```python
from build123d import *

# Parameters (mm, degrees)
SKETCH_1_R          = 1.6
EXTRUDE_1_DEPTH     = 3
CUT_EXTRUDE_1_DEPTH = 4
SKETCH_4_R          = 43
CUT_EXTRUDE_2_DEPTH = 10
FILLET_1_R          = 2


with BuildPart() as part:
    # 草图1 → 凸台-拉伸1 (new body)
    with BuildSketch(Plane.XY):
        with BuildLine():
            Line((45.024979201, 5), (65, 5))
            Line((65, 5), (65, -5))
            Line((65, -5), (50, -20))
            Line((50, -20), (10, -20))
            Line((10, -20), (-5, -5))
            Line((-5, -5), (-5, 5))
            Line((-5, 5), (14.975020799, 5))
            ThreePointArc((14.975020799, 5), (30, 1.5), (45.024979201, 5))
        make_face()
        with Locations((60, 0)):
            Circle(SKETCH_1_R, mode=Mode.SUBTRACT)
        Circle(SKETCH_1_R, mode=Mode.SUBTRACT)
    extrude(amount=EXTRUDE_1_DEPTH)

    # 草图3 → 切除-拉伸1 (cut, through all)
    with BuildSketch(Plane(origin=(0, 0, 0), x_dir=(-1, 0, 0), z_dir=(0, 0, -1))):
        Polygon((-25, -15.464816242), (-15, -15.464816242), (-6.245134561, -2.961572616), align=None)
        Polygon((-53.754865439, -2.961572616), (-35, -15.464816242), (-45, -15.464816242), align=None)
    extrude(amount=-CUT_EXTRUDE_1_DEPTH, mode=Mode.SUBTRACT)

    # 草图4 → 切除-拉伸2 (cut)
    with BuildSketch(Plane.XY.offset(3)):
        with Locations((30, 35.5)):
            Circle(SKETCH_4_R)
    extrude(amount=-CUT_EXTRUDE_2_DEPTH, mode=Mode.SUBTRACT)

    # 圆角1
    fillet_1_edges = [part.edges().sort_by_distance(p)[0] for p in [
        (50, -20, 1.5),
        (10, -20, 1.5),
        (-5, -5, 1.5),
        (-5, 5, 1.5),
        (65, 5, 1.5),
        (65, -5, 1.5),
        (25, -15.464816242, 1.5),
        (6.245134561, -2.961572616, 1.5),
        (15, -15.464816242, 1.5),
        (45, -15.464816242, 1.5),
        (53.754865439, -2.961572616, 1.5),
        (35, -15.464816242, 1.5),
        (-0.310889132, 5, 1.5),
        (60.310889132, 5, 1.5),
    ]]
    fillet(fillet_1_edges, radius=FILLET_1_R)


solid = part.part
```
The model under review builds one solid part; all positions refer to its coordinate system, in mm. A direction names the side the tool comes from. Give positions to 0.01 mm unless a question says otherwise; leave off trailing zeros. Write each loop counter-clockwise with the first axis right and the second up, starting at its lowest first coordinate (ties: lowest second). Pieces come first, ordered by that corner, then holes. Notation, with made-up numbers: M 16.5,2.25 L 63.5,2.25 A29 cw 63.5,40.25 Z; hole C 49.5,26.25 d9. An arc over 180 degrees is marked long. Write item = value, one per line. Start each with the question number.
Q1. For line 1 (X direction, y = 1, z = 1.9); line 2 (X direction, y = -14.25, z = 2.55); line 3 (X direction, y = -9.5, z = 0.7), list the stretches that pass through material, from the lowest coordinate up.
Q2. We need section A-A (z = 1.6). Give the number of separate pieces and of enclosed holes in the cut face, plus the area to 3 significant figures.
Q3. Clearance check with a flat-ended pin moving along its axis: pin 1 (0.7 mm diameter, centred on x = 43, z = 2, fed in from +Y). State where the tip first meets the part, or that it passes through.
Q4. Machinability: for faces 4 (the face through (30, -10, 3)), 5 (the face through (-0.37, 4.85, 1.52)), 6 (the face through (13.387, -13.161, 1.479)), which of the approach directions +Z, -Z, +X, -X, +Y, -Y give a long, thin tool a straight path to every point of the face, cutting with its end or side? Answer none if there is none.
Q5. We need section C-C (y = -13.25). State the section outline as (x, z) points, plus the area to 3 significant figures.
Q6. We need section D-D (x = 34). State the section outline as (y, z) points, plus the area to 3 significant figures.
Q7. Mouldability with a two-part tool opening along Y and no side actions: class faces 1 (the face through (30, -10, 0)), 2 (the face through (-2, 5, 1)), 3 (the face through (12.578, -9.097, 1.521)) as released by +Y, released by -Y, zero draft, split by the parting line, or undercut.
Q8. We need section B-B (y = 0). State the section outline as (x, z) points.
Result set:
q1.line_1 = -5 to -1.25, 1.25 to 4.33, 55.67 to 58.75, 61.25 to 65
q1.line_2 = 4.25 to 14.15, 20.23 to 39.77, 45.85 to 55.75
q1.line_3 = -0.5 to 12.26, 16.05 to 43.95, 47.74 to 60.5
q2.separate_pieces = 1
q2.enclosed_holes = 4
q2.area = 908 mm2
q3.pin_1 = -5.38
q4.face_4 = +Z, +X, -X, +Y, -Y
q4.face_5 = +Z, -Z, +Y
q4.face_6 = +Z, -Z
q5.outline = M 3.25,0 L 13.45,0 L 13.45,3 L 3.25,3 Z; M 20.38,0 L 39.62,0 L 39.62,3 L 20.38,3 Z; M 46.55,0 L 56.75,0 L 56.75,3 L 46.55,3 Z
q5.area = 119 mm2
q6.outline = M -20,0 L -7.31,0 L -7.31,3 L -20,3 Z
q6.area = 38.1 mm2
q7.face_1 = zero draft
q7.face_2 = released by +Y
q7.face_3 = undercut
q8.outline = M -5,0 L -1.6,0 L -1.6,3 L -5,3 Z; M 1.6,0 L 5.74,0 L 5.74,3 L 1.6,3 Z; M 54.26,0 L 58.4,0 L 58.4,3 L 54.26,3 Z; M 61.6,0 L 65,0 L 65,3 L 61.6,3 Z
